```python
from build123d import *

# Parameters (mm, degrees)
F1_DEPTH = 2
F2_R     = 10.16
F3_R     = 152.4


with BuildPart() as f1:
    # F0 (on Front) → F1 (new body)
    with BuildSketch(Plane.XZ):
        Polygon((-146.152106, 9.9886), (-112.152106, 0), (126.847894, 0), (160.847894, 9.9987), (160.847894, 39.9987), (126.847894, 50), (-112.152106, 50), (-146.152106, 39.986), align=None)
    extrude(amount=F1_DEPTH)

    # F2
    f2_edges = [f1.edges().sort_by_distance(p)[0] for p in [
        (-146.152106, -1, 39.986),
        (-146.152106, -1, 9.9886),
        (160.847894, -1, 9.9987),
        (160.847894, -1, 39.9987),
    ]]
    fillet(f2_edges, radius=F2_R)

    # F3
    f3_edges = [f1.edges().sort_by_distance(p)[0] for p in [
        (126.847894, -1, 50),
        (126.847894, -1, 0),
        (-112.152106, -1, 50),
        (-112.152106, -1, 0),
    ]]
    fillet(f3_edges, radius=F3_R)


solid = f1.part
```
Could you check a few things on this model? Use its own coordinates, in mm. Round coordinates to 2 decimals unless told otherwise and drop trailing zeros. Loops run counter-clockwise (first coordinate to the right, second up) from the corner with the lowest first, then second, coordinate; pieces in that order, holes last. Notation, with made-up numbers: (68, -38) - (115, -38) arc R26 ccw to (115, -24) - close; hole circle Ø4 at (-24, -25). An arc over 180 degrees is marked (long way). Answer in a Markdown table with one row per item. Add a question column.
(1) I'm going to push a flat-ended pin straight in: pin 1 (1 mm diameter, centred on y = -0.5, z = 38, fed in from -X). Where does the tip first touch, or does it pass through?
(2) If we section it at B-B (x = -114): Please give me the cut outline in (y, z), plus the area to 3 significant figures.
(3) I need wall thicknesses on line 1 along Z through (x, y) = (135, -0.25); line 2 along X through (y, z) = (-0.75, 9.5); line 3 along Z through (x, y) = (-122.5, -1.65). Which ranges of each line are inside material? Lowest first, please.
(4) If we section it at A-A (y = -1.7): Please give me the cut outline in (x, z), plus the area to 3 significant figures.
(5) If we section it at C-C (z = 11): Please give me the cut outline in (x, y), plus the area to 3 significant figures.
Model answer:
| question | item | result |
|---|---|---|
| 1 | pin 1 | stops at x = -144.77 |
| 2 | outline | (-2, 1.87) - (0, 1.87) - (0, 48.13) - (-2, 48.13) - close |
| 2 | area | 92.5 mm² |
| 3 | line 1 | z = 3 to 47 |
| 3 | line 2 | x = -142.13 to 156.82 |
| 3 | line 3 | z = 3.46 to 46.53 |
| 4 | outline | (-146.15, 17.59) arc R10.16 ccw to (-138.86, 7.85) - (-133.19, 6.18) arc R152.4 ccw to (-90.23, 0) - (104.9, 0) arc R152.4 ccw to (147.9, 6.19) - (153.55, 7.85) arc R10.16 ccw to (160.85, 17.6) - (160.85, 32.4) arc R10.16 ccw to (153.56, 42.14) - (147.91, 43.81) arc R152.4 ccw to (104.9, 50) - (-90.18, 50) arc R152.4 ccw to (-133.23, 43.79) - (-138.86, 42.13) arc R10.16 ccw to (-146.15, 32.39) - close |
| 4 | area | 14,500 mm² |
| 5 | outline | (-143.72, -2) - (158.41, -2) - (158.41, 0) - (-143.72, 0) - close |
| 5 | area | 604 mm² |
